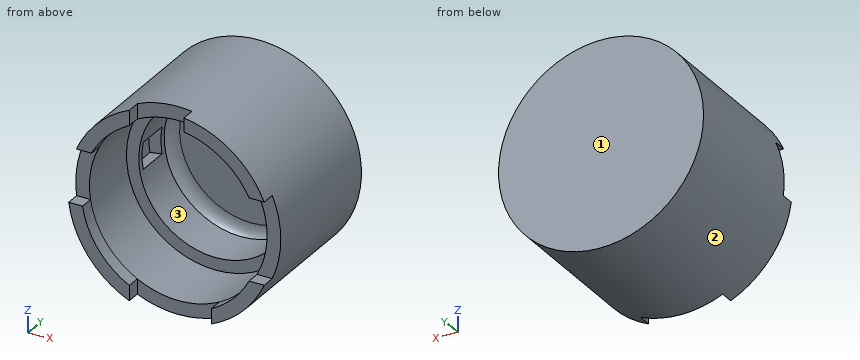
from build123d import *

# Parameters (mm, degrees)
FILLET1_R            = 4.064
SKETCH10_W           = 2.857500069
SKETCH10_H           = 7.5184
REVOLVE3_ANGLE       = 20
CUT_EXTRUDE1_START   = 1.27
CUT_EXTRUDE1_DEPTH   = 4.9784
CIRPATTERN4_COUNT    = 2
FILLET8_R            = 1.27
FILLET9_R            = 1.27
SKETCH13_W           = 23.8125
SKETCH13_H           = 35.179
SKETCH14_OUTSIDE_W   = 64.822
SKETCH14_OUTSIDE_H   = 64.822
SKETCH14_OUTSIDE_W_2 = 18.870013955
SKETCH14_OUTSIDE_H_2 = 18.870013955
SKETCH14_OUTSIDE_W_3 = 25.220013955
SKETCH14_OUTSIDE_H_3 = 25.220013955
CUT_EXTRUDE2_DEPTH   = 3.175


with BuildPart() as part:
    # Sketch1 → Revolve1 (revolve)
    with BuildSketch(Plane.XY, mode=Mode.PRIVATE) as revolve1_sk:
        Polygon((0, 9.1059), (-20.6375, 9.1059), (-20.6375, 5.042647059), (-17.78, 5.042647059), (-17.78, -5.042647059), (-20.6375, -5.042647059), (-20.6375, -19.7231), (-16.51, -19.7231), (-16.51, -15.5956), (-18.0975, -15.5956), (-18.0975, -13.3096), (-16.51, -13.3096), (-16.51, 6.7564), (-3.8481, 6.7564), (-3.0861, 7.5184), (0, 7.5184), align=None)
    revolve(revolve1_sk.sketch.rotate(Axis((0, 0, 0), (0, 1, 0)), 270), axis=Axis((0, 0, 0), (0, 1, 0)))

    # Fillet1
    # the kernel refuses this fillet: 4.064 mm, written as the material it takes off along each edge
    with BuildSketch(Plane(origin=(0, 9.1059, 0), x_dir=(0, 0, -1), z_dir=(1, 0, 0))) as fillet1_piece_1:
        with BuildLine():
            CenterArc((16.573500069, -4.064), FILLET1_R, 0.010532312, 89.989467688)
            Line((20.6375, -4.063252941), (20.718779999, -4.063238))
            Line((20.718779999, -4.063238), (20.71878, 0))
            Line((20.71878, 0), (20.6375, 0.08128))
            Line((20.6375, 0.08128), (16.573500069, 0.08128))
            Line((16.573500069, 0.08128), (16.573500069, 0))
        make_face()
    revolve(axis=Axis((0, 9.1059, 0), (0, 1, 0)), mode=Mode.SUBTRACT)

    # Sketch10 → Revolve3 (revolve, symmetric)
    with BuildSketch(Plane.XY) as revolve3_sk:
        with Locations((-19.208750034, 0)):
            Rectangle(SKETCH10_W, SKETCH10_H)
    revolve3 = revolve(axis=Axis((0, 0, 0), (0, 1, 0)), revolution_arc=REVOLVE3_ANGLE / 2)
    revolve3 = revolve3 + revolve(revolve3_sk.sketch, axis=Axis((0, 0, 0), (0, -1, 0)), revolution_arc=REVOLVE3_ANGLE / 2)

    # Sketch12 → Cut-Extrude1 (cut)
    with BuildSketch(Plane(origin=(0, -3.7592, 0), x_dir=(1, 0, 0), z_dir=(0, 1, 0)).offset(CUT_EXTRUDE1_START)):
        with BuildLine():
            Line((-7.313638514, 0), (-17.215440903, 1.745954919))
            ThreePointArc((-17.215440903, 1.745954919), (-17.30375, 0), (-17.215440903, -1.745954919))
            Line((-17.215440903, -1.745954919), (-7.313638514, 0))
        make_face()
    cut_extrude1 = extrude(amount=CUT_EXTRUDE1_DEPTH, mode=Mode.SUBTRACT)

    # CirPattern4: Revolve3, Cut-Extrude1 ×2 about axis
    cirpattern4_axis = Axis((0, 0, 0), (0, 1, 0))
    add([revolve3.rotate(cirpattern4_axis, i * 360 / CIRPATTERN4_COUNT) for i in range(1, CIRPATTERN4_COUNT)])
    add([cut_extrude1.rotate(cirpattern4_axis, i * 360 / CIRPATTERN4_COUNT) for i in range(1, CIRPATTERN4_COUNT)], mode=Mode.SUBTRACT)

    # Fillet8
    # the kernel refuses this fillet: 1.27 mm, written as the material it takes off along each edge
    with BuildSketch(Plane(origin=(-16.431533746, -2.4892, -1.607730937), x_dir=(0.1324793231915166, 0, -0.9911857691304479), z_dir=(0, 1, 0)), Plane(origin=(16.431533746, -2.4892, 1.607730937), x_dir=(-0.13247932319151873, 0, 0.9911857691304475), z_dir=(0, 1, 0))) as fillet8_piece_1:
        with BuildLine():
            CenterArc((1.211424462, 1.269207194), FILLET8_R, 201.909884157, 66.065503548)
            Line((0.033154154, 0.795309438), (0.009588748, 0.785831483))
            ThreePointArc((0.009588748, 0.785831483), (-0.008800881, 0.398712653), (-0.025377958, 0.001057934))
            Line((-0.025377958, 0.001057934), (0.000897351, -0.025384144))
            ThreePointArc((0.000897351, -0.025384144), (0.583278445, -0.01509352), (1.165659538, -0.025384144))
            Line((1.165659538, -0.025384144), (1.166556889, 0))
        make_face()
    extrude(amount=4.9784, mode=Mode.SUBTRACT)
    with BuildSketch(Plane(origin=(-16.431533746, -2.4892, 1.607730937), x_dir=(0.13247932319152245, 0, 0.9911857691304472), z_dir=(0, 1, 0)), Plane(origin=(16.431533746, -2.4892, -1.607730937), x_dir=(-0.13247932319151992, 0, -0.9911857691304475), z_dir=(0, 1, 0))) as fillet8_piece_2:
        with BuildLine():
            CenterArc((1.211424462, -1.269207194), FILLET8_R, 92.024612295, 66.065503548)
            Line((0.033154154, -0.795309438), (0.009588748, -0.785831483))
            ThreePointArc((0.009588748, -0.785831483), (-0.008800881, -0.398712653), (-0.025377958, -0.001057934))
            Line((-0.025377958, -0.001057934), (0.000897351, 0.025384144))
            ThreePointArc((0.000897351, 0.025384144), (0.583278445, 0.01509352), (1.165659538, 0.025384144))
            Line((1.165659538, 0.025384144), (1.166556889, 0))
        make_face()
    extrude(amount=4.9784, mode=Mode.SUBTRACT)

    # Fillet9
    fillet9_edges = [part.edges().sort_by_distance(p)[0] for p in [
        (-17.215440903, 0, 1.745954919),
        (-17.215440903, 0, -1.745954919),
        (17.215440903, 0, -1.745954919),
        (17.215440903, 0, 1.745954919),
    ]]
    fillet(fillet9_edges, radius=FILLET9_R)


with BuildPart() as body_2:
    # Sketch13 → Revolve4 (revolve)
    with BuildSketch(Plane.XY):
        with Locations((-11.90625, -5.3086)):
            Rectangle(SKETCH13_W, SKETCH13_H)
    revolve(axis=Axis((0, 12.2809, 0), (0, -1, 0)))

    # Intersect1: read off the stored shape, not the designer's step
    # Intersect1: cut part
    add(part.part, mode=Mode.SUBTRACT)

    # Sketch14 outside → Cut-Extrude2 (cut)
    with BuildSketch(Plane.XZ.offset(22.8981)):
        Rectangle(SKETCH14_OUTSIDE_W, SKETCH14_OUTSIDE_H)
        with Locations((-18.960006978, 18.960006978)):
            Rectangle(SKETCH14_OUTSIDE_W_2, SKETCH14_OUTSIDE_H_2, mode=Mode.SUBTRACT)
        with Locations((15.785006978, 18.960006978)):
            Rectangle(SKETCH14_OUTSIDE_W_3, SKETCH14_OUTSIDE_H_2, mode=Mode.SUBTRACT)
        with Locations((-18.960006978, -15.785006978)):
            Rectangle(SKETCH14_OUTSIDE_W_2, SKETCH14_OUTSIDE_H_3, mode=Mode.SUBTRACT)
        with Locations((18.960006978, -18.960006978)):
            Rectangle(SKETCH14_OUTSIDE_W_2, SKETCH14_OUTSIDE_H_2, mode=Mode.SUBTRACT)
    extrude(amount=-CUT_EXTRUDE2_DEPTH, mode=Mode.SUBTRACT)

    # Sketch15 → Cut-Revolve5 (revolve, cut)
    with BuildSketch(Plane.XY):
        Polygon((0, -22.8981), (20.6375, -22.8981), (20.6375, -19.7231), (17.504044696, -19.7231), (17.504044696, -16.22202595), (19.900999595, -16.22202595), (19.900999595, -12.241789307), (17.504044696, -12.241789307), (17.504044696, 7.5184), (0, 7.5184), align=None)
    revolve(axis=Axis((0, 0, 0), (0, -1, 0)), mode=Mode.SUBTRACT)


solid = body_2.part
CAD build for the part. Positions are in the model's coordinates, mm. Face numbers are marked on the shaded views. Coordinates: 2 decimals unless noted, no trailing zeros. Loops run counter-clockwise (first coordinate to the right, second up) from the corner with the lowest first, then second, coordinate; pieces in that order, holes last. Notation, with made-up numbers: (33, 10) - (72, 10) arc R18 ccw to (72, 14) - close; hole circle Ø7 at (-23, 77.5). An arc over 180 degrees is marked (long way). Use one line per item in the form item = value. Start each with the question number.
1) Drill centre lines: L1, parallel to X at y = -9.5, z = 0; L2, parallel to Y at x = -4, z = -1; L3, parallel to X at y = -17, z = -15. Where is each one in solid material? Low to high. Write a range as from..to.
2) Flat gauge pins, fed straight in: pin 1 (1 mm diameter, centred on x = -14.5, y = 5, fed in from -Z); pin 2 (4 mm diameter, centred on x = -7, y = -7.5, fed in from -Z); pin 3 (1.5 mm diameter, centred on x = -1, z = 7.5, fed in from -Y). Where does each tip first touch, or does it go through?
3) Two-plate mould, pull along Z, no slides. Class the marked faces 1, 2 and 3: +Z half, -Z half, draft (parallel to the pull), parting line (faces both ways), or undercut.
4) Band-saw the part on D-D (y = -15). Give the cut face in (x, z) (1 decimal), and give its area (3 significant figures).
5) Band-saw the part on B-B (y = 3). Give the cut face in (x, z) (1 decimal), and give its area (3 significant figures).
6) Band-saw the part on A-A (z = 0). Give the cut face in (x, y), and give its area (3 significant figures).
7) Band-saw the part on C-C (x = 0). Give the cut face in (y, z), and give its area (3 significant figures).
Check values:
q1.L1 = -23.81..-20.64, 20.64..23.81
q1.L2 = 9.11..12.28
q1.L3 = -18.49..-14.17, 14.17..18.49
q2.pin_1 = -19.26
q2.pin_2 = -23.28
q2.pin_3 = 9.11
q3.face_1 = draft
q3.face_2 = parting line
q3.face_3 = undercut
q4.outline = circle Ø47.6 at (0, 0); hole circle Ø41.3 at (0, 0)
q4.area = 443 mm2
q5.outline = circle Ø47.6 at (0, 0); hole (-20.3, -3.6) - (-17.5, -3.1) arc R17.8 ccw to (17.5, -3.1) - (20.3, -3.6) arc R20.6 ccw to (20.3, 3.6) - (17.5, 3.1) arc R17.8 ccw to (-17.5, 3.1) - (-20.3, 3.6) arc R20.6 ccw to start
q5.area = 750 mm2
q6.outline = (-23.81, -19.72) - (-20.64, -19.72) - (-20.64, -5.04) - (-17.78, -5.04) - (-17.78, -3.76) - (-20.64, -3.76) - (-20.64, 3.76) - (-17.78, 3.76) - (-17.78, 5.04) - (-20.64, 5.04) arc R4.06 cw to (-16.57, 9.11) - (16.57, 9.11) arc R4.06 cw to (20.64, 5.04) - (17.78, 5.04) - (17.78, 3.76) - (20.64, 3.76) - (20.64, -3.76) - (17.78, -3.76) - (17.78, -5.04) - (20.64, -5.04) - (20.64, -19.72) - (23.81, -19.72) - (23.81, 12.28) - (-23.81, 12.28) - close
q6.area = 356 mm2
q7.outline = (-19.72, -23.81) - (12.28, -23.81) - (12.28, 23.81) - (-19.72, 23.81) - (-19.72, 20.64) - (-5.04, 20.64) - (-5.04, 17.78) - (5.04, 17.78) - (5.04, 20.64) arc R4.06 cw to (9.11, 16.57) - (9.11, -16.57) arc R4.06 cw to (5.04, -20.64) - (5.04, -17.78) - (-5.04, -17.78) - (-5.04, -20.64) - (-19.72, -20.64) - close
q7.area = 399 mm2
